Drawing for the job (mm, zero at the part's lowest x, y, z). Give positions to 0.01 mm unless a question says otherwise; leave off trailing zeros. Loops run counter-clockwise (first coordinate to the right, second up) from the corner with the lowest first, then second, coordinate; pieces in that order, holes last. Notation, with made-up numbers: (32, -12) -> (62, -12) arc R9 ccw to (62, -5) -> close; hole circle Ø7 at (57.25, 57.25). An arc over 180 degrees is marked (long way). Answer in a Markdown table with one row per item. Add a question column.
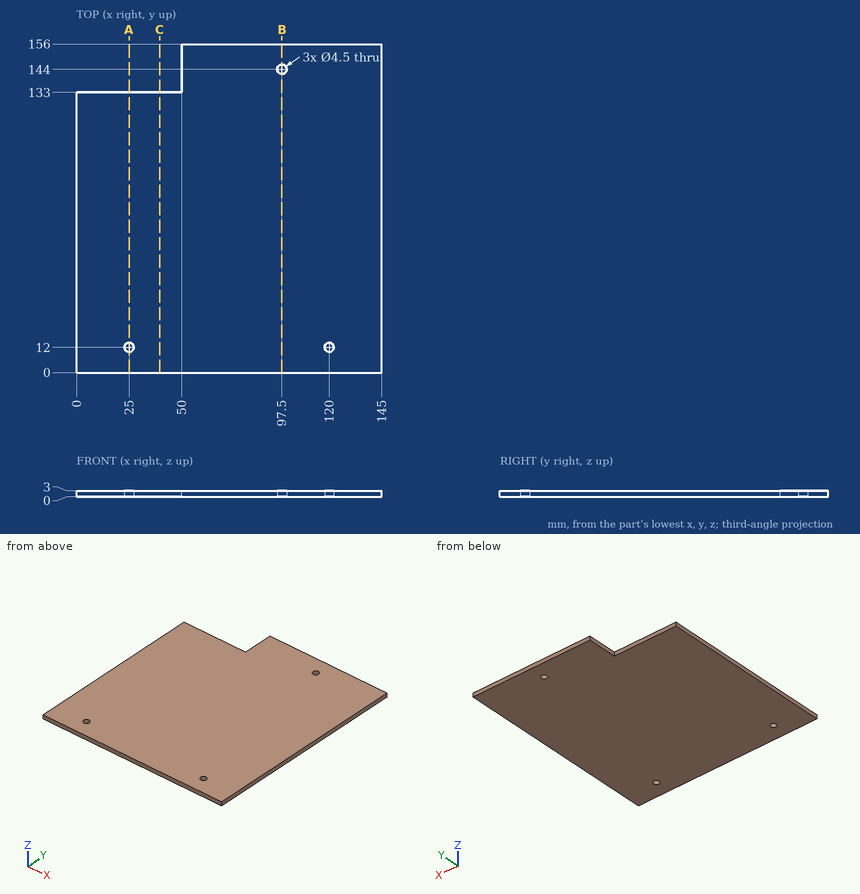
(1) Wall check: line 1 along X through (y, z) = (12, 1); line 2 along Y through (x, z) = (97.5, 2.1); line 3 along Y through (x, z) = (120, 2.2). Give the ranges that are in metal, low to high. Write a range as from..to.
(2) Saw through at B-B, the plane x = 97.5. List the corners of the cut face in (y, z), then the cut area to 4 significant figures.
(3) Saw through at C-C, the plane x = 39.5. List the corners of the cut face in (y, z), then the cut area to 3 significant figures.
(4) Saw through at A-A, the plane x = 25. List the corners of the cut face in (y, z).
(5) Flat gauge pin, fed straight in: pin 1 Ø1.5 at (x, z) = (17, 0.5) entering from +Y. Where does the tip first touch, or does it go through?
Worked answers:
| question | item | result |
|---|---|---|
| 1 | line 1 | 0..22.75, 27.25..117.75, 122.25..145 |
| 1 | line 2 | 0..141.75, 146.25..156 |
| 1 | line 3 | 0..9.75, 14.25..156 |
| 2 | outline | (0, 0) -> (141.75, 0) -> (141.75, 3) -> (0, 3) -> close; (146.25, 0) -> (156, 0) -> (156, 3) -> (146.25, 3) -> close |
| 2 | area | 454.5 mm^2 |
| 3 | outline | (0, 0) -> (133, 0) -> (133, 3) -> (0, 3) -> close |
| 3 | area | 399 mm^2 |
| 4 | outline | (0, 0) -> (9.75, 0) -> (9.75, 3) -> (0, 3) -> close; (14.25, 0) -> (133, 0) -> (133, 3) -> (14.25, 3) -> close |
| 5 | pin 1 | y = 133 |
